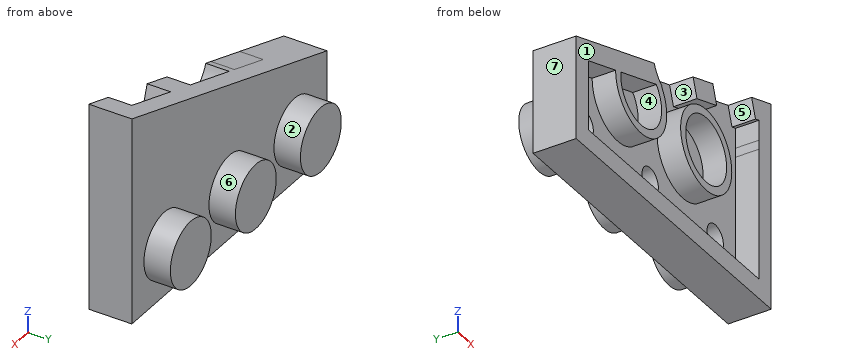
Autodesk Inventor part; units mm, degrees
ref_plane "YZ Plane" through (0, 0, 0) normal (1, 0, 0) x (0, 1, 0)
ref_plane "XZ Plane" through (0, 0, 0) normal (0, 1, 0) x (-1, 0, 0)
ref_plane "XY Plane" through (0, 0, 0) normal (0, 0, 1) x (1, 0, 0)
sketch "Sketch1" plane through (0, 0, 0) normal (0, 1, 0) x (-1, 0, 0)
  line L0 (0, 0) -> (0, 15.5956)
  line L1 (0, 0) -> (23.3934, 0)
  line L2 (23.3934, 0) -> (23.3934, 7.7978)
  line L3 (23.3934, 7.7978) -> (0, 15.5956)
  dimension "d0" = 15.5956
  dimension "d1" = 23.3934
  dimension "d2" = 7.7978
extrude "Extrusion1" add sketch "Sketch1" along normal blind 3.236
sketch "Sketch2" plane through (0, 3.236, 0) normal (0, 1, 0) x (1, 0, 0)
  line L0 (-23.3934, -7.7978) -> (0, -15.5956)
  line L1 (-23.3934, 0) -> (-23.3934, -7.7978)
  line L2 (0, 0) -> (-23.3934, 0)
  line L3 (-23.3934, 0) -> (-23.3934, -7.7978)
  circle A0 centre (-19.4945, -3.8989) radius 2.4498
  line L4 (-23.3934, 0) -> (-19.4945, 0) construction
  line L5 (-19.4945, 0) -> (-19.4945, -3.8989) construction
  line L6 (-19.4945, -3.8989) -> (-23.3934, -3.8989) construction
  line L7 (-23.3934, -3.8989) -> (-23.3934, 0) construction
  dimension "d7" = 4.8997
  dimension "d17" = 3.8989
  dimension "d18" = 3.8989
extrude "Extrusion2" add sketch "Sketch2" along normal blind 1.9837
pattern_linear "Rectangular Pattern1" count 3 spacing 7.7978 along (1, 0, 0) of "Extrusion2"
sketch "Sketch3" plane through (0, 0, 0) normal (0, -1, 0) x (1, 0, 0)
  point P0 (0, 0)
shell "Shell1" thickness 1.4732 removed faces 1 at (-7.7978, 0, 7.7978)
sketch "Sketch4" plane through (-21.9202, 1.7628, 1.4732) normal (0, -1, 0) x (1, 0, 0)
  circle A0 centre (18.0213, 2.4257) radius 0.9766 construction
  circle A1 centre (10.2235, 2.4257) radius 0.9766 construction
  circle A2 centre (2.4257, 2.4257) radius 0.9766 construction
  line L0 (20.447, 12.0784) -> (20.447, 0)
  line L1 (0, 5.2628) -> (20.447, 12.0784)
  line L2 (0, 0) -> (0, 5.2628) construction
  line L3 (20.447, 0) -> (0, 0) construction
  circle A3 centre (18.0213, 2.4257) radius 2.4498 construction
  circle A4 centre (10.2235, 2.4257) radius 0.9766 construction
  circle A5 centre (10.2235, 2.4257) radius 2.4498 construction
  circle A6 centre (2.4257, 2.4257) radius 2.4498 construction
  line L4 (18.0213, 2.4257) -> (10.2235, 2.4257) construction
  line L5 (10.2235, 2.4257) -> (2.4257, 2.4257) construction
  line L6 (18.0213, 2.4257) -> (18.0213, 10.2235) construction
  line L7 (18.0213, 2.4257) -> (25.8191, 2.4257) construction
  line L8 (18.0213, 10.2235) -> (10.2235, 2.4257) construction
  circle A7 centre (14.1224, 6.3246) radius 3.064
  circle A8 centre (14.1224, 6.3246) radius 2.4498
  point P0 (21.9202, -1.4732)
  dimension "d14" = 7.7978
  dimension "d15" = 90
  dimension "d16" = 4.8997
extrude "Extrusion3" add sketch "Sketch4" along normal up to surface (1.7628 mm away)
pattern_linear "Rectangular Pattern2" count 2 spacing 7.7978 along (-1, 0, 0) of "Extrusion3"
sketch "Sketch5" plane through (-21.9202, 1.7628, 1.4732) normal (0, -1, 0) x (1, 0, 0)
  circle A0 centre (18.0213, 2.4257) radius 2.4498 construction
  line L0 (18.0213, 2.4257) -> (18.0213, 10.2235) construction
  line L1 (18.0213, 2.4257) -> (25.8191, 2.4257) construction
  circle A1 centre (18.0213, 10.2235) radius 2.4498 construction
  circle A2 centre (14.1224, 6.3246) radius 3.064 construction
  line L2 (15.6972, 9.4488) -> (13.6906, 15.4684) construction
  line L3 (13.6906, 15.4684) -> (19.2087, 14.4083) construction
  line L4 (19.2087, 14.4083) -> (20.3454, 10.9982) construction
  line L5 (21.9202, 14.1224) -> (7.2702, 9.2391) construction
  arc A3 (15.6972, 9.4488) -> (20.3454, 10.9982) centre (18.0213, 10.2235) ccw
  line L6 (20.3454, 10.9982) -> (19.2087, 14.4083)
  line L7 (15.6972, 9.4488) -> (13.6906, 15.4684)
  line L8 (13.6906, 15.4684) -> (19.2087, 14.4083)
  circle A4 centre (10.2235, 2.4257) radius 2.4498 construction
  line L9 (10.2235, 2.4257) -> (10.2235, 10.2235) construction
  line L10 (10.2235, 2.4257) -> (18.0213, 2.4257) construction
  circle A5 centre (10.2235, 10.2235) radius 2.4498 construction
  line L11 (13.4213, 8.3773) -> (11.5486, 13.9952) construction
  line L12 (11.5486, 13.9952) -> (1.2037, 10.5468) construction
  line L13 (1.2037, 10.5468) -> (2.2026, 7.5499) construction
  line L14 (3.8194, 8.0888) -> (-1.4732, 6.3246) construction
  line L15 (2.2026, 7.5499) -> (7.8994, 9.4488) construction
  arc A6 (13.1382, 9.2263) -> (11.9558, 8.4912) centre (14.1224, 6.3246) ccw construction
  arc A7 (13.1382, 9.2263) -> (11.9558, 8.4912) centre (14.1224, 6.3246) ccw
  arc A8 (7.8994, 9.4488) -> (11.9558, 8.4912) centre (10.2235, 10.2235) ccw
  line L16 (13.1382, 9.2263) -> (11.5486, 13.9952)
  line L17 (11.5486, 13.9952) -> (1.2037, 10.5468)
  line L18 (1.2037, 10.5468) -> (2.2026, 7.5499)
  line L19 (2.2026, 7.5499) -> (7.8994, 9.4488)
  point P0 (21.9202, -1.4732)
  dimension "d24" = 7.7978
  dimension "d25" = 90
  dimension "d28" = 7.7978
  dimension "d29" = 90
extrude "Extrusion4" cut sketch "Sketch5" along normal up to surface (1.7628 mm away)
properties part number "other diagonal piece" material "ABS Plastic"
Can you work these out from the model? Positions are in its coordinate system, mm. Face numbers are marked on the shaded views. A direction names the side the tool comes from. Coordinates: 2 decimals unless noted, no trailing zeros. Loops run counter-clockwise (first coordinate to the right, second up) from the corner with the lowest first, then second, coordinate; pieces in that order, holes last. Notation, with made-up numbers: M 23,56 L 50,56 A7 ccw 50,66 Z; hole C 25.25,51.5 d11. An arc over 180 degrees is marked long. Return JSON: item names as keys, results as strings. Group by question number.
Item 1: I'm going to push flat-ended pins straight in: pin 1 Ø0.6 at (x, z) = (-11.5, 4.5) entering from -Y; pin 2 Ø1.3 at (x, z) = (-17, 10) entering from +Y; pin 3 Ø1.2 at (y, z) = (0.5, 12.5) entering from -X. Where does each tip first touch, or does it pass through?
Item 2: On a 3-axis mill with a long thin cutter (end or side, diameter ignored), from which of +Z, -Z, +X, -X, +Y, -Y can I reach the whole of each face in a straight line? I mean the marked faces 1, 2, 3 and 4. Say none if no direction works.
Item 3: Imagine slicing it at B-B (y = 2.65). Please give me the cut outline in (x, z), and give its area (3 significant figures).
Item 4: Thinking about a two-plate mould opening in Z: for the marked faces 5, 6 and 7, which applies, released by +Z, released by -Z, zero draft, split by the parting line, or undercut?
Item 5: Imagine slicing it at A-A (y = 1.3). Give the number of separate pieces and of enclosed holes in the cut face, and give its area (3 significant figures).
Item 6: Imagine slicing it at C-C (z = 8.5). Please give me the cut outline in (x, y).
Item 7: If I drill on L1, parallel to X at y = 3.15, z = 3.75; L2, parallel to Z at x = -15, y = 0.5; L3, parallel to X at y = 1.5, z = 3.5, over which ranges is the centre line in solid material (lowest first)? Write a range as from..to.
Item 8: Imagine slicing it at D-D (x = -11.5). Please give me the cut outline in (y, z).
Verdict:
{
 "1": {"pin 1": "stops at y = 3.75", "pin 2": "stops at y = 3.24", "pin 3": "stops at x = -9.37"},
 "2": {"face 1": "+Z, -Z, +X, -X, -Y", "face 2": "+Y", "face 3": "-X, -Y", "face 4": "-Y"},
 "3": {"outline": "M -23.39,0 L 0,0 L 0,15.6 L -23.39,7.8 Z; hole C -19.49,3.9 d1.95; hole C -11.7,3.9 d1.95; hole C -3.9,3.9 d1.95", "area": "265 mm^2"},
 "4": {"face 5": "undercut", "face 6": "split by the parting line", "face 7": "zero draft"},
 "5": {"separate pieces": "3", "enclosed holes": "2", "area": "99.3 mm^2"},
 "6": {"outline": "M -21.29,0 L -16.63,0 L -16.63,1.76 L -13.25,1.76 L -13.25,0 L -12.61,0 L -12.61,1.76 L -10.78,1.76 L -10.78,0 L -10.14,0 L -10.14,1.76 L -5.45,1.76 L -5.45,0 L -4.82,0 L -4.82,1.76 L -1.47,1.76 L -1.47,0 L 0,0 L 0,3.24 L -21.29,3.24 Z"},
 "7": {"L1": "x = -23.39..-20.46, -18.53..-12.66, -10.73..-4.86, -2.93..0", "L2": "z = 0..1.47, 4.79..5.42, 9.04..10.6", "L3": "x = -23.39..-21.92, -1.47..0"},
 "8": {"outline": "M 0,0 L 3.24,0 L 3.24,1.46 L 5.22,1.46 L 5.22,6.34 L 3.24,6.34 L 3.24,11.76 L 1.76,11.76 L 1.76,4.86 L 3.75,4.86 L 3.75,2.94 L 1.76,2.94 L 1.76,1.47 L 0,1.47 Z"}
}
